from build123d import *

# Parameters (mm, degrees)
BOSS_EXTRUDE1_DEPTH = 4
SKETCH2_W           = 191
SKETCH2_H           = 5
CUT_EXTRUDE1_DEPTH  = 2.5


with BuildPart() as part:
    # Sketch1 → Boss-Extrude1 (new body)
    with BuildSketch(Plane(origin=(0, 0, 0), x_dir=(1, 0, 0), z_dir=(0, 1, 0))):
        Polygon((-70, 70), (-70, 65.5), (-50, 65.5), (-50, 70), (-30, 70), (-30, 65.5), (-10, 65.5), (-10, 70), (10, 70), (10, 65.5), (30, 65.5), (30, 70), (50, 70), (50, 65.5), (70, 65.5), (70, 70), (90, 70), (90, 65.5), (100, 65.5), (100, 51), (95.5, 51), (95.5, 36.5), (100, 36.5), (100, 22), (95.5, 22), (95.5, 7.5), (100, 7.5), (100, -7), (95.5, -7), (95.5, -21.5), (100, -21.5), (100, -36), (95.5, -36), (95.5, -50.5), (100, -50.5), (100, -65.5), (90, -65.5), (90, -70), (70, -70), (70, -65.5), (50, -65.5), (50, -70), (30, -70), (30, -65.5), (10, -65.5), (10, -70), (-10, -70), (-10, -65.5), (-30, -65.5), (-30, -70), (-50, -70), (-50, -65.5), (-70, -65.5), (-70, -70), (-90, -70), (-90, -65.5), (-100, -65.5), (-100, -50.5), (-95.5, -50.5), (-95.5, -36), (-100, -36), (-100, -21.5), (-95.5, -21.5), (-95.5, -7), (-100, -7), (-100, 7.5), (-95.5, 7.5), (-95.5, 22), (-100, 22), (-100, 36.5), (-95.5, 36.5), (-95.5, 51), (-100, 51), (-100, 65.5), (-90, 65.5), (-90, 70), align=None)
    extrude(amount=BOSS_EXTRUDE1_DEPTH)

    # Sketch2 → Cut-Extrude1 (cut)
    with BuildSketch(Plane(origin=(0, 4, 0), x_dir=(1, 0, 0), z_dir=(0, 1, 0))):
        with Locations((0, 58)):
            Rectangle(SKETCH2_W, SKETCH2_H)
        with Locations((0, -58)):
            Rectangle(SKETCH2_W, SKETCH2_H)
    extrude(amount=-CUT_EXTRUDE1_DEPTH, mode=Mode.SUBTRACT)


solid = part.part
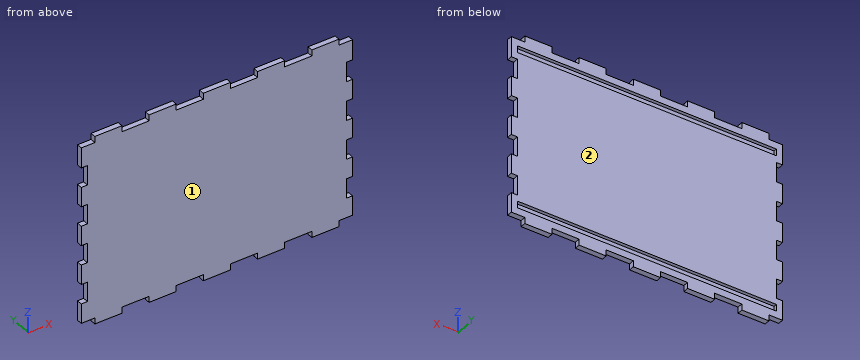
Model file for the job. Use its own axes, mm. Face numbers are marked on the shaded views. Give positions to 0.01 mm unless a question says otherwise; leave off trailing zeros. Loops run counter-clockwise (first coordinate to the right, second up) from the corner with the lowest first, then second, coordinate; pieces in that order, holes last.
1) Wall check: line 1 (Z direction, x = -83, y = 2.7); line 2 (Z direction, x = -64.5, y = 2.65); line 3 (X direction, y = 3.8, z = -57). Give the ranges that are in metal, low to high.
2) Saw through at C-C (y = 2.25). Count the separate pieces of the cut face and the enclosed holes in it, plus the area to 3 significant figures.
3) Saw through at D-D (x = 15). Write the cut outline in (y, z).
4) Flat gauge pins, fed straight in: pin 1 Ø1.5 at (y, z) = (3.5, -43) entering from +X; pin 2 Ø1.2 at (x, y) = (98, 1.5) entering from +Z; pin 3 Ø1.2 at (x, y) = (-55, 2) entering from -Z. Where does each tip first touch, or does it go through?
5) Saw through at A-A (x = -84). Write the cut outline in (y, z).
6) Pull direction Y, two halves, no side cores. Call the marked faces 1 and 2: +Y half, -Y half, draft (parallel to the pull), parting line (faces both ways), or undercut.
7) Saw through at B-B (z = 19.5). Write the cut outline in (x, y), plus the area to 3 significant figures.
Answer block:
1. line 1: z = -70 to -60.5, -55.5 to 55.5, 60.5 to 70
1. line 2: z = -65.5 to -60.5, -55.5 to 55.5, 60.5 to 65.5
1. line 3: x = -100 to -95.5, 95.5 to 100
2. separate pieces: 1
2. enclosed holes: 2
2. area: 24,700 mm2
3. outline: (0, -65.5) - (4, -65.5) - (4, -60.5) - (1.5, -60.5) - (1.5, -55.5) - (4, -55.5) - (4, 55.5) - (1.5, 55.5) - (1.5, 60.5) - (4, 60.5) - (4, 65.5) - (0, 65.5) - close
4. pin 1: stops at x = 95.5
4. pin 2: stops at z = 65.5
4. pin 3: stops at z = -65.5
5. outline: (0, -70) - (4, -70) - (4, -60.5) - (1.5, -60.5) - (1.5, -55.5) - (4, -55.5) - (4, 55.5) - (1.5, 55.5) - (1.5, 60.5) - (4, 60.5) - (4, 70) - (0, 70) - close
6. face 1: -Y half
6. face 2: +Y half
7. outline: (-95.5, 0) - (95.5, 0) - (95.5, 4) - (-95.5, 4) - close
7. area: 764 mm2
